Check sheet for the modelled part. Datum: model origin and axes. Units: mm. A direction names the side the tool comes from. Give positions to 0.01 mm unless a question says otherwise; leave off trailing zeros. Loops run counter-clockwise (first coordinate to the right, second up) from the corner with the lowest first, then second, coordinate; pieces in that order, holes last.
```python
from build123d import *

# Parameters (mm, degrees)
SKETCH1_R           = 2.25
BOSS_EXTRUDE1_DEPTH = 56.2
SHELL1_T            = -1.5
SKETCH2_W           = 107.526504688
SKETCH2_H           = 43.658783516
CUT_EXTRUDE1_DEPTH  = 54.7
FILLET1_R           = 1.5
SKETCH3_R           = 10
CUT_EXTRUDE2_DEPTH  = 123.692467131
SKETCH4_R           = 10
CUT_EXTRUDE3_DEPTH  = 167.248879786
SKETCH6_W           = 22.5
SKETCH6_H           = 15
CUT_EXTRUDE5_DEPTH  = 0.25


with BuildPart() as part:
    # Sketch1 → Boss-Extrude1 (new body)
    with BuildSketch(Plane(origin=(0, 0, 0), x_dir=(1, 0, 0), z_dir=(0, 1, 0))):
        with BuildLine():
            Line((-70.193094701, 34.5), (69.806905299, 34.5))
            ThreePointArc((69.806905299, 34.5), (73.342439205, 33.035533906), (74.806905299, 29.5))
            Line((74.806905299, 29.5), (74.806905299, -39.5))
            ThreePointArc((74.806905299, -39.5), (73.342439205, -43.035533906), (69.806905299, -44.5))
            Line((69.806905299, -44.5), (-70.193094701, -44.5))
            ThreePointArc((-70.193094701, -44.5), (-73.728628607, -43.035533906), (-75.193094701, -39.5))
            Line((-75.193094701, -39.5), (-75.193094701, 29.5))
            ThreePointArc((-75.193094701, 29.5), (-73.728628607, 33.035533906), (-70.193094701, 34.5))
        make_face()
        with Locations(Location((68.5, 28.35, 0), (0, 0, 270))):
            Circle(SKETCH1_R, mode=Mode.SUBTRACT)
        with Locations(Location((68.5, -38.35, 0), (0, 0, 270))):
            Circle(SKETCH1_R, mode=Mode.SUBTRACT)
        with Locations(Location((-68.5, -38.35, 0), (0, 0, 90))):
            Circle(SKETCH1_R, mode=Mode.SUBTRACT)
        with Locations(Location((-68.5, 28.35, 0), (0, 0, 90))):
            Circle(SKETCH1_R, mode=Mode.SUBTRACT)
        with BuildLine():
            Line((-34.6, 11.135640978), (-34.6, 12.25))
            Line((-34.6, 12.25), (-31.4, 12.25))
            Line((-31.4, 12.25), (-31.4, 11.135640978))
            ThreePointArc((-31.4, 11.135640978), (-33, -11.25), (-34.6, 11.135640978))
        make_face(mode=Mode.SUBTRACT)
        with BuildLine():
            Line((-1.6, 11.135640978), (-1.6, 12.25))
            Line((-1.6, 12.25), (1.6, 12.25))
            Line((1.6, 12.25), (1.6, 11.135640978))
            ThreePointArc((1.6, 11.135640978), (0, -11.25), (-1.6, 11.135640978))
        make_face(mode=Mode.SUBTRACT)
        with BuildLine():
            Line((38.4, 11.135640978), (38.4, 12.25))
            Line((38.4, 12.25), (41.6, 12.25))
            Line((41.6, 12.25), (41.6, 11.135640978))
            ThreePointArc((41.6, 11.135640978), (40, -11.25), (38.4, 11.135640978))
        make_face(mode=Mode.SUBTRACT)
    extrude(amount=BOSS_EXTRUDE1_DEPTH)

    # Shell1
    shell1_openings = [part.faces().sort_by_distance(p)[0] for p in [
        (-0.193094701, 56.2, -32.804682921),
    ]]
    offset(amount=SHELL1_T, openings=shell1_openings, kind=Kind.INTERSECTION)

    # Sketch2 → Cut-Extrude1 (cut)
    with BuildSketch(Plane(origin=(0, 56.2, 0), x_dir=(1, 0, 0), z_dir=(0, 1, 0))):
        Rectangle(SKETCH2_W, SKETCH2_H)
    extrude(amount=-CUT_EXTRUDE1_DEPTH, mode=Mode.SUBTRACT)

    # Fillet1
    fillet1_edges = [part.edges().sort_by_distance(p)[0] for p in [
        (-75.193094701, 0, 5),
        (-73.728628607, 0, -33.035533906),
        (-0.193094701, 0, -34.5),
        (73.342439205, 0, -33.035533906),
        (74.806905299, 0, 5),
        (73.342439205, 0, 43.035533906),
        (-0.193094701, 0, 44.5),
        (-73.728628607, 0, 43.035533906),
    ]]
    fillet(fillet1_edges, radius=FILLET1_R)

    # Sketch3 → Cut-Extrude2 (cut, through all)
    with BuildSketch(Plane(origin=(0, 0, -34.5), x_dir=(-1, 0, 0), z_dir=(0, 0, -1))):
        with Locations((0.129531499, 37.7)):
            Circle(SKETCH3_R)
    extrude(amount=-CUT_EXTRUDE2_DEPTH, mode=Mode.SUBTRACT)

    # Sketch4 → Cut-Extrude3 (cut, through all)
    with BuildSketch(Plane.ZY.offset(75.193094701)):
        with Locations((5, 37.7)):
            Circle(SKETCH4_R)
    extrude(amount=-CUT_EXTRUDE3_DEPTH, mode=Mode.SUBTRACT)

    # Sketch6 → Cut-Extrude5 (cut)
    with BuildSketch(Plane.XZ):
        with Locations((-33, 30.85)):
            Rectangle(SKETCH6_W, SKETCH6_H)
        with Locations((40, 30.85)):
            Rectangle(SKETCH6_W, SKETCH6_H)
        with Locations((0, 30.85)):
            Rectangle(SKETCH6_W, SKETCH6_H)
    extrude(amount=-CUT_EXTRUDE5_DEPTH, mode=Mode.SUBTRACT)


solid = part.part
```
(1) Gauge pin test, flat ends, axial feed: pin 1 Ø12 at (x, z) = (1.5, 30.5) entering from -Y; pin 2 Ø0.9 at (y, z) = (0.5, -12) entering from +X; pin 3 Ø0.6 at (y, z) = (1, -12) entering from -X. Record the tip position at first contact, or that the pin passes through.
(2) Access from +Z, -Z, +X, -X, +Y, -Y to the whole of each face (thin tool, end or side, straight path). Record for faces 5 (the face through (73.303, 28.467, -33.074)), 6 (the face through (71.66, 28.47, -26.33)).
(3) Section check D-D on x = 5. Record the boundary of the cut face in (y, z).
(4) Section check A-A on y = 21. Give the number of separate pieces and of enclosed holes in the cut face, plus the area to 3 significant figures.
(5) Section check B-B on x = 40. Record the boundary of the cut face in (y, z), plus the area to 3 significant figures.
(6) Material ranges on line 1 (Z direction, x = 57, y = 41); line 2 (X direction, y = 25, z = 16); line 3 (X direction, y = 12, z = -28.35), recorded low to high.
(7) Section check C-C on z = 32. Record the boundary of the cut face in (x, y).
(8) Release check for a two-part mould opening along Y. For faces 1 (the face through (40, 0.25, 31)), 2 (the face through (-72.64, 28.47, 42)), 3 (the face through (1.172, 47.615, 43.74)), 4 (the face through (-1, 1.5, 13)) record: pulls with the +Y half, pulls with the -Y half, needs draft (parallel to the pull), parting line crosses it, or undercut.
Computed values:
1. pin 1: stops at y = 0.25
1. pin 2: stops at x = 74.7
1. pin 3: stops at x = -75.18
2. face 5: -Z, +X, +Y, -Y
2. face 6: +Y
3. outline: (0, -33) arc R1.5 ccw to (1.5, -34.5) - (29.12, -34.5) - (29.12, -33) - (1.5, -33) - (1.5, -10.08) - (0, -10.08) - close; (0, 10.08) - (1.5, 10.08) - (1.5, 43) - (29.12, 43) - (29.12, 44.5) - (1.5, 44.5) arc R1.5 ccw to (0, 43) - (0, 38.35) - (0.25, 38.35) - (0.25, 23.35) - (0, 23.35) - close; (46.28, -34.5) - (56.2, -34.5) - (56.2, -33) - (46.28, -33) - close; (46.28, 43) - (56.2, 43) - (56.2, 44.5) - (46.28, 44.5) - close
4. separate pieces: 5
4. enclosed holes: 5
4. area: 780 mm2
5. outline: (0, -33) arc R1.5 ccw to (1.5, -34.5) - (56.2, -34.5) - (56.2, -33) - (1.5, -33) - (1.5, -12.25) - (0, -12.25) - close; (0, 11.25) - (1.5, 11.25) - (1.5, 43) - (56.2, 43) - (56.2, 44.5) - (1.5, 44.5) arc R1.5 ccw to (0, 43) - (0, 38.35) - (0.25, 38.35) - (0.25, 23.35) - (0, 23.35) - close
5. area: 243 mm2
6. line 1: z = -34.5 to -33, 43 to 44.5
6. line 2: x = -75.19 to -73.69, 73.31 to 74.81
6. line 3: x = -75.19 to -73.69, -72.25 to -70.75, -66.25 to -64.75, 64.75 to 66.25, 70.75 to 72.25, 73.31 to 74.81
7. outline: (-75.19, 1.5) arc R1.5 ccw to (-73.69, 0) - (-44.25, 0) - (-44.25, 0.25) - (-21.75, 0.25) - (-21.75, 0) - (-11.25, 0) - (-11.25, 0.25) - (11.25, 0.25) - (11.25, 0) - (28.75, 0) - (28.75, 0.25) - (51.25, 0.25) - (51.25, 0) - (73.31, 0) arc R1.5 ccw to (74.81, 1.5) - (74.81, 56.2) - (73.31, 56.2) - (73.31, 1.5) - (-73.69, 1.5) - (-73.69, 56.2) - (-75.19, 56.2) - close
8. face 1: pulls with the -Y half
8. face 2: needs draft
8. face 3: undercut
8. face 4: pulls with the +Y half
